Could you check a few things on this model? Use its own coordinates, in mm. A direction names the side the tool comes from. Give positions to 0.01 mm unless a question says otherwise; leave off trailing zeros. Loops run counter-clockwise (first coordinate to the right, second up) from the corner with the lowest first, then second, coordinate; pieces in that order, holes last.
1. Imagine slicing it at D-D (z = -3). List the corners of the cut face in (x, y) for me.
2. Imagine slicing it at C-C (y = -0.9). Count the separate pieces of the cut face and the enclosed holes in it, plus the area to 3 significant figures.
3. For P1, Ø1.5, axis at y = 1, z = 18, coming from the +X side; P2, Ø3.5, axis at x = 33.24, z = 13.42, coming from the +Y side; P3, Ø5, axis at x = 39.39, z = -11.77, coming from the +Y side; P4, Ø2, axis at y = 1, z = -31.5, coming from the +X side, each with a flat end and sliding along its axis, tell me the tip position at first contact or that it passes through.
4. I need wall thicknesses on line 1 along Z through (x, y) = (-8, 1); line 2 along X through (y, z) = (1.6, -11); line 3 along X through (y, z) = (-0.9, 40). Which ranges of each line are inside material? Lowest first, please.
5. Thinking about a two-plate mould opening in X: for faces 3 (the cylindrical face through (-30.492, -0.028, -30.135)), 4 (the flat face through (-43.1, 0.03, -25.35)), 5 (the flat face through (12, -2, -12)), which applies, +X half, -X half, draft (parallel to the pull), parting line (faces both ways), or undercut?
6. For faces 1 (the flat face through (12, 2, -12)), 2 (the flat face through (26.5, 0, 15.1)), which set-ups out of +Z, -Z, +X, -X, +Y, -Y let a thin tool reach every point of the face, with its end or its side?
7. Imagine slicing it at B-B (x = 17.5). List the corners of the cut face in (y, z) for me.
8. Imagine slicing it at A-A (z = 40). List the corners of the cut face in (x, y) for me, plus the area to 3 significant figures.
```python
from build123d import *

# Parameters (mm, degrees)
SKETCH1_R           = 2
BOSS_EXTRUDE1_DEPTH = 2
SKETCH3_R           = 2
CUT_EXTRUDE1_DEPTH  = 10
FILLET1_R           = 1


with BuildPart() as part:
    # Sketch1 → Boss-Extrude1 (new, symmetric)
    with BuildSketch(Plane(origin=(0, 0, 0), x_dir=(1, 0, 0), z_dir=(0, 1, 0))):
        Polygon((-28.867513459, 50), (-57.735026919, 0), (-28.867513459, -50), (28.867513459, -50), (57.735026919, 0), (28.867513459, 50), align=None)
        with Locations(Location((29.891016151, 28.227241336, 0), (0, 0, 270))):
            Circle(SKETCH1_R, mode=Mode.SUBTRACT)
        with Locations(Location((39.391016151, 11.772758664, 0), (0, 0, 270))):
            Circle(SKETCH1_R, mode=Mode.SUBTRACT)
        with Locations(Location((-9.5, -40, 0), (0, 0, 270))):
            Circle(SKETCH1_R, mode=Mode.SUBTRACT)
        with Locations(Location((9.5, -40, 0), (0, 0, 270))):
            Circle(SKETCH1_R, mode=Mode.SUBTRACT)
        with Locations(Location((-39.391016151, 11.772758664, 0), (0, 0, 90))):
            Circle(SKETCH1_R, mode=Mode.SUBTRACT)
        with Locations(Location((-29.891016151, 28.227241336, 0), (0, 0, 90))):
            Circle(SKETCH1_R, mode=Mode.SUBTRACT)
    extrude(amount=BOSS_EXTRUDE1_DEPTH, both=True)

    # Sketch3 → Cut-Extrude1 (cut)
    with BuildSketch(Plane(origin=(0, 2, 0), x_dir=(1, 0, 0), z_dir=(0, 1, 0))):
        with Locations(Location((-10.490381057, 11.830127019, 0), (0, 0, 270))):
            Circle(SKETCH3_R)
        with Locations(Location((33.243901834, -13.419872981, 0), (0, 0, 270))):
            Circle(SKETCH3_R)
        with Locations(Location((28.243901834, -22.080127019, 0), (0, 0, 270))):
            Circle(SKETCH3_R)
        with Locations(Location((-15.490381057, 3.169872981, 0), (0, 0, 270))):
            Circle(SKETCH3_R)
        Polygon((-13.660254038, -3.660254038), (-3.660254038, 13.660254038), (31.413774815, -6.589745962), (21.413774815, -23.910254038), align=None)
    extrude(amount=-CUT_EXTRUDE1_DEPTH, mode=Mode.SUBTRACT)

    # Fillet1
    fillet1_edges = [part.edges().sort_by_distance(p)[0] for p in [
        (21.413774815, 0, 23.910254038),
        (-13.660254038, 0, 3.660254038),
        (-3.660254038, 0, -13.660254038),
        (31.413774815, 0, 6.589745962),
    ]]
    fillet(fillet1_edges, radius=FILLET1_R)


solid = part.part
```
Derived:
1. outline: (-56, -2) - (-17.48, -2) - (-17.48, 2) - (-56, 2) - close; (-13.5, -2) - (-9.81, -2) - (-9.81, 2) - (-13.5, 2) - close; (14.8, -2) - (56, -2) - (56, 2) - (14.8, 2) - close
2. separate pieces: 1
2. enclosed holes: 11
2. area: 7,730 mm2
3. P1: stops at x = 47.78
3. P2: passes through
3. P3: stops at y = 2
3. P4: stops at x = 40.13
4. line 1: z = -50 to -6.14, 6.93 to 38.68, 41.32 to 50
4. line 2: x = -51.38 to -41.24, -37.55 to -12.31, -8.67 to -5.2, 0.95 to 37.55, 41.24 to 51.38
4. line 3: x = -34.64 to -11.5, -7.5 to 7.5, 11.5 to 34.64
5. face 3: undercut
5. face 4: -X half
5. face 5: draft
6. face 1: +Z, -Z, +X, -X, +Y
6. face 2: +Y, -Y
7. outline: (-2, -50) - (2, -50) - (2, -1.44) - (-2, -1.44) - close; (-2, 21.65) - (2, 21.65) - (2, 50) - (-2, 50) - close
8. outline: (-34.64, -2) - (-11.5, -2) - (-11.5, 2) - (-34.64, 2) - close; (-7.5, -2) - (7.5, -2) - (7.5, 2) - (-7.5, 2) - close; (11.5, -2) - (34.64, -2) - (34.64, 2) - (11.5, 2) - close
8. area: 245 mm2
